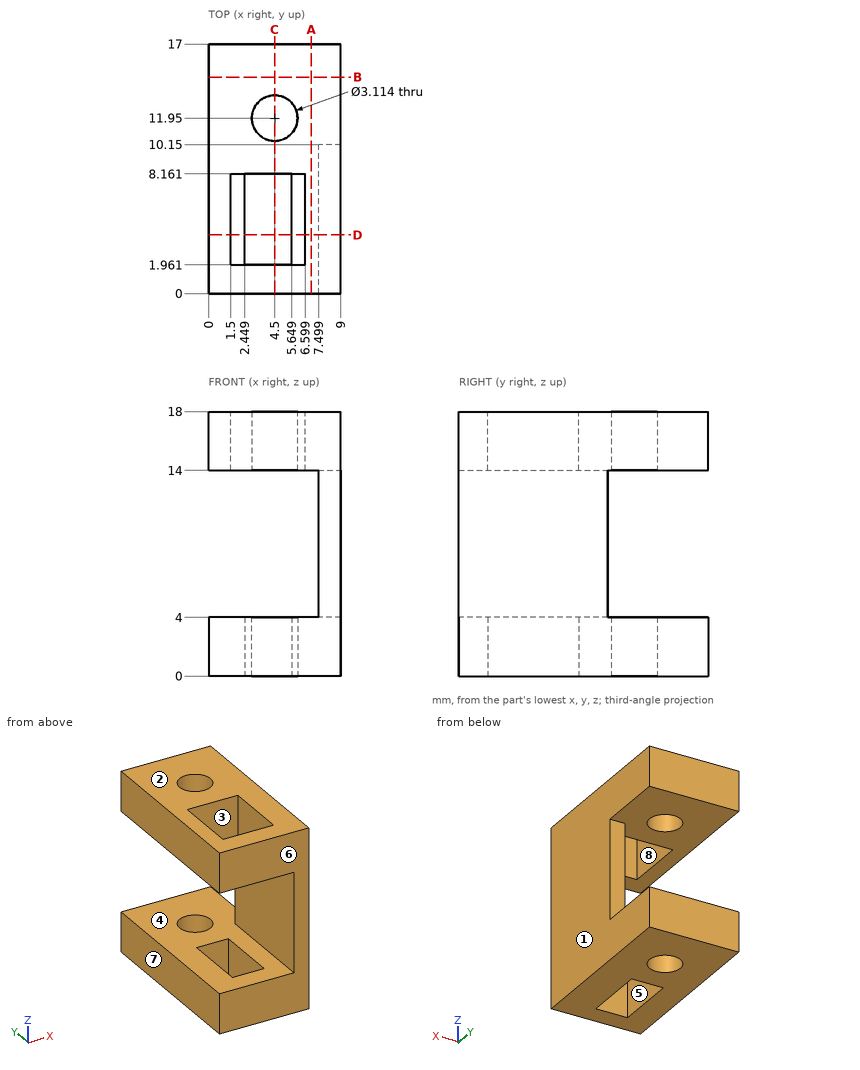
Answer from the drawing. Dimensions are ordinates in mm from the lowest x, y and z of the part. A direction names the side the tool comes from. Give positions to 0.01 mm unless a question says otherwise; leave off trailing zeros. Order: outer loops, then holes, each group sorted by start corner. A loop starts at its lowest first (then second) coordinate and runs counter-clockwise, first axis right, second up. Notation, with made-up numbers: (6.5, 50.5) - (52.5, 50.5) arc R30 cw to (52.5, 81.5) - close; hole circle Ø10 at (9.5, -34.5). An arc over 180 degrees is marked (long way). One line per item, written item: value. Start each with the question number.
1. Consider line 1 (Y direction, x = 4.5, z = 1.55); line 2 (Z direction, x = 3.25, y = 14.75); line 3 (X direction, y = 5.25, z = 1.25). Determine where each line is inside the solid, lowest interval first.
2. Section B-B, the plane y = 14.75 is taken. Write down the section's boundary in (x, z).
3. This flat-tipped pin is pushed along its axis until it touches: pin 1 Ø0.8 at (x, z) = (8, 9) entering from +Y. Where does it stop, or does it pass through?
4. Which of the six approach directions +Z, -Z, +X, -X, +Y, -Y give full straight-line access (tool end or side, diameter ignored) to the marked faces 1, 2, 3, 4 and 5?
5. Section D-D, the plane y = 4 is taken. Write down the section's boundary in (x, z).
6. For a pull along X with two mould halves and no side action, classify the marked faces 6, 7 and 8 as released by +X, released by -X, zero draft, split by the parting line, or undercut.
7. Section A-A, the plane x = 7 is taken. Write down the section's boundary in (y, z), then the cut area to 3 significant figures.
8. Section C-C, the plane x = 4.5 is taken. Write down the section's boundary in (y, z).
Filled sheet:
1. line 1: 0 to 1.96, 8.16 to 10.39, 13.51 to 17
1. line 2: 0 to 4, 14 to 18
1. line 3: 0 to 2.45, 5.65 to 9
2. outline: (0, 0) - (9, 0) - (9, 4) - (0, 4) - close; (0, 14) - (9, 14) - (9, 18) - (0, 18) - close
3. pin 1: y = 10.15
4. face 1: +Z, -Z, +X, +Y, -Y
4. face 2: +Z, +X, -X, +Y, -Y
4. face 3: +Z
4. face 4: -X, +Y
4. face 5: +Z, -Z
5. outline: (0, 0) - (2.45, 0) - (2.45, 4) - (0, 4) - close; (0, 14) - (1.5, 14) - (1.5, 18) - (0, 18) - close; (5.65, 0) - (9, 0) - (9, 18) - (6.6, 18) - (6.6, 14) - (7.5, 14) - (7.5, 4) - (5.65, 4) - close
6. face 6: zero draft
6. face 7: released by -X
6. face 8: undercut
7. outline: (0, 0) - (17, 0) - (17, 4) - (0, 4) - close; (0, 14) - (17, 14) - (17, 18) - (0, 18) - close
7. area: 136 mm²
8. outline: (0, 0) - (1.96, 0) - (1.96, 4) - (0, 4) - close; (0, 14) - (1.96, 14) - (1.96, 18) - (0, 18) - close; (8.16, 0) - (10.39, 0) - (10.39, 4) - (8.16, 4) - close; (8.16, 14) - (10.39, 14) - (10.39, 18) - (8.16, 18) - close; (13.51, 0) - (17, 0) - (17, 4) - (13.51, 4) - close; (13.51, 14) - (17, 14) - (17, 18) - (13.51, 18) - close
